Could you check a few things on this model? Use its own coordinates, in mm. Give positions to 0.01 mm unless a question says otherwise; leave off trailing zeros. Loops run counter-clockwise (first coordinate to the right, second up) from the corner with the lowest first, then second, coordinate; pieces in that order, holes last. Notation, with made-up numbers: (75.5, 48) - (92.5, 48) arc R16 ccw to (92.5, 71) - close; hole circle Ø5 at (-19, -33.5). An arc over 180 degrees is marked (long way). Write each question's results on one line, items separated by ' | '. Start each with the question number.
(1) I need wall thicknesses on line 1 (X direction, y = 8, z = 12.7); line 2 (Z direction, x = 0.25, y = -9); line 3 (Z direction, x = 9.75, y = -6). Which ranges of each line are inside material? Lowest first, please.
(2) Suppose I cut it at B-B (x = 2.75). Please give me the cut outline in (y, z) (3 decimals), and give its area (3 significant figures).
(3) For pin 1 (5 mm diameter, centred on y = 2, z = 18, fed in from +X), with a flat end and sliding along its axis, tell me the tip position at first contact or that it passes through.
(4) Suppose I cut it at A-A (z = 12.7). Please give me the cut outline in (x, y) (3 decimals).
(5) Suppose I cut it at C-C (y = -5.25). Please give me the cut outline in (x, z) (3 decimals).
(6) If we mould it in two halves opening along X, with no side actions, what happens to faces 1 (the face through (-4.27, 9.32, 8.02)), 2 (the face through (0, 12.573, 6)), 3 (the face through (-11.772, -11.872, 12.833)), 4 (the face through (-4.27, -9.69, 8.02))? For each: released by +X, released by -X, zero draft, split by the parting line, or undercut.
(7) Suppose I cut it at D-D (z = 2.75). Please give me the cut outline in (x, y).
Autodesk Inventor part; units mm, degrees
ref_plane "YZ Plane" through (0, 0, 0) normal (1, 0, 0) x (0, 1, 0)
ref_plane "XZ Plane" through (0, 0, 0) normal (0, 1, 0) x (-1, 0, 0)
ref_plane "XY Plane" through (0, 0, 0) normal (0, 0, 1) x (1, 0, 0)
sketch "Sketch1" plane through (0, 0, 0) normal (0, 0, 1) x (1, 0, 0)
  line L0 (-12.677, 12.5729) -> (12.723, 12.5729)
  line L1 (12.723, 12.5729) -> (12.723, -12.8271)
  line L2 (12.723, -12.8271) -> (-12.677, -12.8271)
  line L3 (-12.677, -12.8271) -> (-12.677, 12.5729)
  point P0 (0, 0)
  dimension "d0" = 25.4
  dimension "d1" = 25.4
extrude "Extrusion1" add sketch "Sketch1" along normal blind 25.4
fillet "Fillet1" radius 3.175 12 edges at (0.023, 12.5729, 0) (-12.677, 12.5729, 12.7) (0.023, 12.5729, 25.4) (12.723, 12.5729, 12.7) (12.723, -0.1271, 0) (12.723, -0.1271, 25.4) (12.723, -12.8271, 12.7) (-12.677, -0.1271, 25.4) (0.023, -12.8271, 25.4) (0.023, -12.8271, 0) (-12.677, -0.1271, 0) (-12.677, -12.8271, 12.7)
hole "Hole1" at (0.023, 12.5729, 12.7) direction (0, -1, 0) diameter 12.7 end through all both
hole "Hole2" at (0.023, -0.1271, 0) direction (0, 0, 1) diameter 12.7 end through all
hole "Hole3" at (-12.677, -0.1271, 12.7) direction (1, 0, 0) diameter 12.7 end through all
properties part number "FirstPart"
Output values:
1) line 1: -12.68 to -6.33, 6.37 to 12.72 | line 2: 0 to 6.35, 19.05 to 25.4 | line 3: 0.01 to 10.29, 15.11 to 25.39
2) outline: (-12.827, 3.175) arc R3.175 ccw to (-9.652, 0) - (-5.862, 0) - (-5.862, 6.965) - (-12.827, 6.965) - close; (-12.827, 18.435) - (-5.862, 18.435) - (-5.862, 25.4) - (-9.652, 25.4) arc R3.175 ccw to (-12.827, 22.225) - close; (5.608, 0) - (9.398, 0) arc R3.175 ccw to (12.573, 3.175) - (12.573, 6.965) - (5.608, 6.965) - close; (5.608, 18.435) - (12.573, 18.435) - (12.573, 22.225) arc R3.175 ccw to (9.398, 25.4) - (5.608, 25.4) - close | area: 185 mm2
3) pin 1: x = 12.72
4) outline: (-12.677, -9.652) arc R3.175 ccw to (-9.502, -12.827) - (-6.327, -12.827) - (-6.327, -6.477) - (-12.677, -6.477) - close; (-12.677, 6.223) - (-6.327, 6.223) - (-6.327, 12.573) - (-9.502, 12.573) arc R3.175 ccw to (-12.677, 9.398) - close; (6.373, -12.827) - (9.548, -12.827) arc R3.175 ccw to (12.723, -9.652) - (12.723, -6.477) - (6.373, -6.477) - close; (6.373, 6.223) - (12.723, 6.223) - (12.723, 9.398) arc R3.175 ccw to (9.548, 12.573) - (6.373, 12.573) - close
5) outline: (-12.677, 3.175) arc R3.175 ccw to (-9.502, 0) - (-3.729, 0) - (-3.729, 7.577) arc R6.35 cw to (-5.1, 8.948) - (-12.677, 8.948) - close; (-12.677, 16.452) - (-5.1, 16.452) arc R6.35 cw to (-3.729, 17.823) - (-3.729, 25.4) - (-9.502, 25.4) arc R3.175 ccw to (-12.677, 22.225) - close; (3.775, 0) - (9.548, 0) arc R3.175 ccw to (12.723, 3.175) - (12.723, 8.948) - (5.146, 8.948) arc R6.35 cw to (3.775, 7.577) - close; (3.775, 17.823) arc R6.35 cw to (5.146, 16.452) - (12.723, 16.452) - (12.723, 22.225) arc R3.175 ccw to (9.548, 25.4) - (3.775, 25.4) - close
6) face 1: undercut | face 2: zero draft | face 3: released by -X | face 4: undercut
7) outline: (-12.65, -9.65) arc R3.15 ccw to (-9.5, -12.8) - (9.55, -12.8) arc R3.15 ccw to (12.69, -9.65) - (12.69, 9.4) arc R3.15 ccw to (9.55, 12.54) - (-9.5, 12.54) arc R3.15 ccw to (-12.65, 9.4) - close; hole circle Ø12.7 at (0.02, -0.13)
